CAD build for the part. Positions are in the model's coordinates, mm. A direction names the side the tool comes from. Round coordinates to 2 decimals unless told otherwise and drop trailing zeros. Loops run counter-clockwise (first coordinate to the right, second up) from the corner with the lowest first, then second, coordinate; pieces in that order, holes last. Notation, with made-up numbers: (7, 62.5) -> (63, 62.5) arc R7 cw to (63, 70.5) -> close; hole circle Ø10 at (-36.75, 58.25). An arc over 180 degrees is marked (long way). Answer as CSV lines item,"result".
```python
from build123d import *

# Parameters (mm, degrees)
ESQUISSE1_R                        = 65
BOSS_EXTRU_1_DEPTH                 = 4
ENL_V_MAT_EXTRU_1_DEPTH            = 93.010868923
BOSS_EXTRU_2_START                 = 12
BOSS_EXTRU_2_DEPTH                 = 12
ENL_V_MAT_EXTRU_2_REACH            = 98.856
ESQUISSE4_R                        = 1.5
CHANFREIN1_SIZE                    = 2
ENL_V_MAT_EXTRU_3_REACH            = 94.704
CONG_1_R                           = 3
ENL_V_MAT_EXTRU_4_DEPTH            = 2
ENL_V_MAT_EXTRU_5_REACH            = 94.984
ESQUISSE8_R                        = 4
R_P_TITION_CIRCULAIRE1_COUNT       = 6
CONG_1_OF_R_P_TITION_CIRCULAIRE1_R = 3


with BuildPart() as part:
    # Esquisse1 → Boss.-Extru.1 (new body)
    with BuildSketch(Plane.XY):
        Circle(ESQUISSE1_R)
    extrude(amount=BOSS_EXTRU_1_DEPTH)

    # Esquisse2 → Enl_v. mat.-Extru.1 (cut, through all)
    with BuildSketch(Plane.XY.offset(4)):
        with BuildLine():
            Line((-2, 1.738533865), (-2, -1.738533865))
            ThreePointArc((-2, -1.738533865), (2.65, 0), (-2, 1.738533865))
        make_face()
    extrude(amount=-ENL_V_MAT_EXTRU_1_DEPTH, mode=Mode.SUBTRACT)

    # Esquisse3 → Boss.-Extru.2 (add)
    with BuildSketch(Plane.XY.offset(4).offset(BOSS_EXTRU_2_START)):
        with BuildLine():
            Line((-5, 2.631064423), (-5, -2.631064423))
            ThreePointArc((-5, -2.631064423), (5.65, 0), (-5, 2.631064423))
        make_face()
        with BuildLine():
            Line((-2, 1.738533865), (-2, -1.738533865))
            ThreePointArc((-2, -1.738533865), (2.65, 0), (-2, 1.738533865))
        make_face(mode=Mode.SUBTRACT)
    extrude(amount=-BOSS_EXTRU_2_DEPTH)

    # Esquisse4 → Enl_v. mat.-Extru.2 (cut, up to next)
    with BuildSketch(Plane.ZY.offset(5), mode=Mode.PRIVATE) as enl_v_mat_extru_2_sk1:
        with Locations((10, 0)):
            Circle(ESQUISSE4_R)
    enl_v_mat_extru_2_tool1 = extrude(enl_v_mat_extru_2_sk1.sketch, amount=-ENL_V_MAT_EXTRU_2_REACH, mode=Mode.PRIVATE) & part.part
    add(enl_v_mat_extru_2_tool1.solids().sort_by_distance((-5, 0, 10))[0], mode=Mode.SUBTRACT)

    # Chanfrein1
    chanfrein1_edges = [part.edges().sort_by_distance(p)[0] for p in [
        (5.65, 0, 4),
        (-5, 0, 4),
    ]]
    chamfer(chanfrein1_edges, length=CHANFREIN1_SIZE)

    # Esquisse5 → Enl_v. mat.-Extru.3 (cut, up to next)
    with BuildSketch(Plane.XY.offset(4), mode=Mode.PRIVATE) as enl_v_mat_extru_3_sk1:
        with BuildLine():
            Line((14.095389312, -5.13030215), (46.984631039, -17.101007166))
            ThreePointArc((46.984631039, -17.101007166), (38.302222156, -32.139380484), (25, -43.301270189))
            Line((25, -43.301270189), (7.5, -12.990381057))
            ThreePointArc((7.5, -12.990381057), (11.490666647, -9.641814145), (14.095389312, -5.13030215))
        make_face()
    enl_v_mat_extru_3_tool1 = extrude(enl_v_mat_extru_3_sk1.sketch, amount=-ENL_V_MAT_EXTRU_3_REACH, mode=Mode.PRIVATE) & part.part
    enl_v_mat_extru_3 = enl_v_mat_extru_3_tool1.solids().sort_by_distance((26.751521, -22.447191, 4))[0]
    add(enl_v_mat_extru_3, mode=Mode.SUBTRACT)

    # Cong_1
    cong_1_edges = [part.edges().sort_by_distance(p)[0] for p in [
        (7.5, -12.990381057, 2),
        (14.095389312, -5.13030215, 2),
        (46.984631039, -17.101007166, 2),
        (25, -43.301270189, 2),
    ]]
    fillet(cong_1_edges, radius=CONG_1_R)

    # Esquisse7 → Enl_v. mat.-Extru.4 (cut)
    with BuildSketch(Plane.XY.offset(4)):
        Polygon((61.058080687, -10.766187015), (58.510776745, -3.767526956), (51.176107371, -2.47422685), (46.388741937, -8.179586805), (48.936045879, -15.178246864), (56.270715253, -16.47154697), align=None)
    enl_v_mat_extru_4 = extrude(amount=-ENL_V_MAT_EXTRU_4_DEPTH, mode=Mode.SUBTRACT)

    # Esquisse8 → Enl_v. mat.-Extru.5 (cut, up to next)
    with BuildSketch(Plane.XY.offset(2), mode=Mode.PRIVATE) as enl_v_mat_extru_5_sk1:
        with Locations((53.723411312, -9.47288691)):
            Circle(ESQUISSE8_R)
    enl_v_mat_extru_5_tool1 = extrude(enl_v_mat_extru_5_sk1.sketch, amount=-ENL_V_MAT_EXTRU_5_REACH, mode=Mode.PRIVATE) & part.part
    enl_v_mat_extru_5 = enl_v_mat_extru_5_tool1.solids().sort_by_distance((53.723411, -9.472887, 2))[0]
    add(enl_v_mat_extru_5, mode=Mode.SUBTRACT)

    # R_p_tition circulaire1: Enl_v. mat.-Extru.3, Enl_v. mat.-Extru.4, Enl_v. mat.-Extru.5 ×6 about axis
    r_p_tition_circulaire1_axis = Axis((0, 0, 0), (0, 0, 1))
    add([enl_v_mat_extru_3.rotate(r_p_tition_circulaire1_axis, i * 360 / R_P_TITION_CIRCULAIRE1_COUNT) for i in range(1, R_P_TITION_CIRCULAIRE1_COUNT)], mode=Mode.SUBTRACT)
    add([enl_v_mat_extru_4.rotate(r_p_tition_circulaire1_axis, i * 360 / R_P_TITION_CIRCULAIRE1_COUNT) for i in range(1, R_P_TITION_CIRCULAIRE1_COUNT)], mode=Mode.SUBTRACT)
    add([enl_v_mat_extru_5.rotate(r_p_tition_circulaire1_axis, i * 360 / R_P_TITION_CIRCULAIRE1_COUNT) for i in range(1, R_P_TITION_CIRCULAIRE1_COUNT)], mode=Mode.SUBTRACT)

    # Cong_1 of R_p_tition circulaire1
    cong_1_of_r_p_tition_circulaire1_edges = [part.edges().sort_by_distance(p)[0] for p in [
        (15, 0, 2),
        (11.490666647, 9.641814145, 2),
        (38.302222156, 32.139380484, 2),
        (50, 0, 2),
        (7.5, 12.990381057, 2),
        (-2.604722665, 14.772116295, 2),
        (-8.682408883, 49.240387651, 2),
        (25, 43.301270189, 2),
        (-7.5, 12.990381057, 2),
        (-14.095389312, 5.13030215, 2),
        (-46.984631039, 17.101007166, 2),
        (-25, 43.301270189, 2),
        (-15, 0, 2),
        (-11.490666647, -9.641814145, 2),
        (-38.302222156, -32.139380484, 2),
        (-50, 0, 2),
        (-7.5, -12.990381057, 2),
        (2.604722665, -14.772116295, 2),
        (8.682408883, -49.240387651, 2),
        (-25, -43.301270189, 2),
    ]]
    fillet(cong_1_of_r_p_tition_circulaire1_edges, radius=CONG_1_OF_R_P_TITION_CIRCULAIRE1_R)


solid = part.part
```
Q1. Drop flat-ended pins along their axis: pin 1 Ø15.5 at (x, y) = (38.5, 42.5) entering from +Z; pin 2 Ø4 at (y, z) = (0, 11.5) entering from -X; pin 3 Ø1 at (x, y) = (5, 4.5) entering from +Z; pin 4 Ø6 at (x, y) = (0, 0) entering from +Z. Give the stop position or say it passes through.
Results:
pin 1,"z = 4"
pin 2,"x = -5"
pin 3,"z = 5.42"
pin 4,"z = 16"
Q2. Slice it at A-A, the plane z = 10. Give the cut face in (x, y).
Results:
outline,"(-5, -2.63) arc R5.65 ccw (long way) to (-5, 2.63) -> (-5, 1.5) -> (-2, 1.5) -> (-2, 1.74) arc R2.65 cw (long way) to (-2, -1.74) -> (-2, -1.5) -> (-5, -1.5) -> close"
Q3. Tool access for faces 3 (the flat face through (-58.63, 13.66, 3.01)), 4 (the cylindrical face through (-14.11, -5.09, 2.03)): list every direction of +Z, -Z, +X, -X, +Y, -Y with a clear straight run to the whole face (end or side of a thin tool).
Results:
face 3,"+Z"
face 4,"+Z, -Z"
Q4. Probe L1, parallel to X at y = -41, z = 1.25; L2, parallel to Y at x = -24.5, z = 1.5; L3, parallel to X at y = -51, z = 1. List the from-to ranges inside material, lowest first. Write a range as [from, to].
Results:
L1,"[-50.44, -38.99], [-31.14, -23.64], [7.23, 23.71], [28.62, 50.44]"
L2,"[-60.21, -20.56], [0, 8.92], [41.69, 60.21]"
L3,"[-40.3, 14.67], [22.65, 40.3]"
Q5. Two-plate mould, pull along X, no slides. Class faces 1 (the conical face through (5.771, -0.22, 5.875)), 2 (the flat face through (-24.61, -20.65, 2.03)): pulls with the +X half, pulls with the -X half, needs draft (parallel to the pull), parting line crosses it, or undercut.
Results:
face 1,"parting line crosses it"
face 2,"undercut"
